Geometry check sheet. Reference: the model listing, model coordinates, mm. A direction names the side the tool comes from. Give positions to 0.01 mm unless a question says otherwise; leave off trailing zeros. Write each loop counter-clockwise with the first axis right and the second up, starting at its lowest first coordinate (ties: lowest second). Pieces come first, ordered by that corner, then holes.
(1) Tool access check on faces 1 (the flat face through (21, 94.5, -21)), 2 (the flat face through (4, 86, -15)), 3 (the flat face through (18, 96, -21.35)). Record the directions out of +Z, -Z, +X, -X, +Y, -Y that give a thin tool (end or side, any length) a straight path to the whole face; none if there is none.
(2) Mould release check, pull along Z, two halves, no side actions. Record for faces 4 (the flat face through (20.915, 23.348, -3.521)), 5 (the flat face through (3.521, 16.698, -15.112)), 6 (the flat face through (16, 76, -2)), 7 (the flat face through (3.521, 13.348, -15.085)): +Z half, -Z half, draft (parallel to the pull), parting line (faces both ways), or undercut.
(3) Cross-section at C-C (y = 33.5). Record the boundary of the cut face in (x, z), and give its area (3 significant figures).
(4) Thickness scan on line 1 along Y through (x, z) = (18, -1.5); line 2 along Y through (x, z) = (1, -18); line 3 along Y through (x, z) = (20, -7). Record the ranges inside material, lowest first.
(5) Cross-section at B-B (z = -9). Record the boundary of the cut face in (x, y).
(6) Cross-section at A-A (x = 3.5). Record the boundary of the cut face in (y, z).
(7) Depth check by flat-ended pin: P1, Ø3, axis at x = 17.5, y = 58.5, coming from the -Z side. Enter the tip coordinate at first touch or a pass-through.
(8) Cross-section at D-D (x = 9). Record the boundary of the cut face in (y, z).
```python
from build123d import *

# Parameters (mm, degrees)
RESSALTO_EXTRUS_O1_DEPTH          = 99.5
FURO_COM_FOLGA_DE_M43_D           = 4.5
FURO_COM_FOLGA_DE_M43_ON_FACE_2_D = 4.5
NERVURA4_START                    = -5
NERVURA4_OUTLINE_W                = 26
NERVURA4_OUTLINE_H                = 26
NERVURA4_DEPTH                    = 5
CORTE_EXTRUS_O3_DEPTH             = 3
CORTE_EXTRUS_O4_DEPTH             = 3
FURO_COM_FOLGA_DE_M42_D           = 4.5
FURO_COM_FOLGA_DE_M42_CSINK_D     = 4.85
FURO_COM_FOLGA_DE_M42_CSINK_ANGLE = 90
CORTE_EXTRUS_O5_DEPTH             = 3
CORTE_EXTRUS_O6_DEPTH             = 3


# Read off the part's stored shape, not the designer's step: Nervura4
with BuildPart() as part:
    # Esboço1 → Ressalto-extrusão1 (new body)
    with BuildSketch(Plane(origin=(0, 0, 0), x_dir=(1, 0, 0), z_dir=(0, 1, 0))):
        Polygon((0, 0), (31, 0), (31, 5), (5, 5), (5, 31), (0, 31), align=None)
    extrude(amount=RESSALTO_EXTRUS_O1_DEPTH)

    # Furo com folga de M43 (through all)
    with Locations(Plane(origin=(0, 84.5, -18), x_dir=(0, 0, -1), z_dir=(-1, 0, 0))):
        with Locations((0, 0), (0, 69.5)):
            Hole(FURO_COM_FOLGA_DE_M43_D / 2)

    # Furo com folga de M43 on face 2 (through all)
    with Locations(Plane(origin=(18, 74.5, 0), x_dir=(1, 0, 0), z_dir=(0, 0, 1))):
        with Locations((0, 0), (0, -49.5)):
            Hole(FURO_COM_FOLGA_DE_M43_ON_FACE_2_D / 2)

    # Nervura4 outline → Nervura4 (add)
    with BuildSketch(Plane(origin=(0, 99.5, 0), x_dir=(1, 0, 0), z_dir=(0, 1, 0)).offset(NERVURA4_START)):
        with Locations((18, 18)):
            Rectangle(NERVURA4_OUTLINE_W, NERVURA4_OUTLINE_H)
    nervura4 = extrude(amount=NERVURA4_DEPTH)

    # Esboço17 → Corte-extrusão3 (cut)
    with BuildSketch(Plane(origin=(0, 0, -5), x_dir=(-1, 0, 0), z_dir=(0, 0, -1))):
        Polygon((-16.065876598, 77.85), (-19.934123402, 77.85), (-21.868246804, 74.5), (-19.934123402, 71.15), (-16.065876598, 71.15), (-14.131753196, 74.5), align=None)
        Polygon((-14.131753196, 25), (-16.065876598, 28.35), (-19.934123402, 28.35), (-21.868246804, 25), (-19.934123402, 21.65), (-16.065876598, 21.65), align=None)
    extrude(amount=-CORTE_EXTRUS_O3_DEPTH, mode=Mode.SUBTRACT)

    # Esboço18 → Corte-extrusão4 (cut)
    with BuildSketch(Plane(origin=(5, 0, 0), x_dir=(0, 0, -1), z_dir=(1, 0, 0))):
        Polygon((19.934123402, 87.85), (16.065876598, 87.85), (14.131753196, 84.5), (16.065876598, 81.15), (19.934123402, 81.15), (21.868246804, 84.5), align=None)
        Polygon((21.868246804, 15), (19.934123402, 18.35), (16.065876598, 18.35), (14.131753196, 15), (16.065876598, 11.65), (19.934123402, 11.65), align=None)
    extrude(amount=-CORTE_EXTRUS_O4_DEPTH, mode=Mode.SUBTRACT)

    # Espelhar1: Nervura4 across plane
    add(nervura4.mirror(Plane(origin=(0, 49.75, 0), x_dir=(0, 0, 1), z_dir=(0, -1, 0))))

    # Furo com folga de M42 (through all)
    with Locations(Plane(origin=(0, 99.5, 0), x_dir=(1, 0, 0), z_dir=(0, 1, 0))):
        with Locations((18, 18)):
            CounterSinkHole(FURO_COM_FOLGA_DE_M42_D / 2, FURO_COM_FOLGA_DE_M42_CSINK_D / 2, counter_sink_angle=FURO_COM_FOLGA_DE_M42_CSINK_ANGLE)

    # Esboço27 → Corte-extrusão5 (cut)
    with BuildSketch(Plane.XZ.offset(-94.5)):
        Polygon((21.868246804, -18), (19.934123402, -14.65), (16.065876598, -14.65), (14.131753196, -18), (16.065876598, -21.35), (19.934123402, -21.35), align=None)
    extrude(amount=-CORTE_EXTRUS_O5_DEPTH, mode=Mode.SUBTRACT)

    # Esboço28 → Corte-extrusão6 (cut)
    with BuildSketch(Plane(origin=(0, 5, 0), x_dir=(1, 0, 0), z_dir=(0, 1, 0))):
        Polygon((19.934123402, 21.35), (16.065876598, 21.35), (14.131753196, 18), (16.065876598, 14.65), (19.934123402, 14.65), (21.868246804, 18), align=None)
    extrude(amount=-CORTE_EXTRUS_O6_DEPTH, mode=Mode.SUBTRACT)


solid = part.part
```
Reply:
1. face 1: -Z, +X
1. face 2: +X
1. face 3: none
2. face 4: draft
2. face 5: undercut
2. face 6: -Z half
2. face 7: undercut
3. outline: (0, -31) - (5, -31) - (5, -5) - (31, -5) - (31, 0) - (0, 0) - close
3. area: 285 mm2
4. line 1: y = 0 to 22.75, 27.25 to 72.25, 76.75 to 99.5
4. line 2: y = 0 to 12.75, 17.25 to 82.25, 86.75 to 99.5
4. line 3: y = 0 to 5, 94.5 to 99.5
5. outline: (0, 0) - (31, 0) - (31, 5) - (5, 5) - (5, 94.5) - (31, 94.5) - (31, 99.5) - (0, 99.5) - close
6. outline: (0, -31) - (99.5, -31) - (99.5, 0) - (0, 0) - close; hole (11.65, -19.93) - (15, -21.87) - (18.35, -19.93) - (18.35, -16.07) - (15, -14.13) - (11.65, -16.07) - close; hole (81.15, -19.93) - (84.5, -21.87) - (87.85, -19.93) - (87.85, -16.07) - (84.5, -14.13) - (81.15, -16.07) - close
7. P1: stops at z = -5
8. outline: (0, -31) - (5, -31) - (5, -5) - (94.5, -5) - (94.5, -31) - (99.5, -31) - (99.5, 0) - (0, 0) - close
